Source: CAD feature listing. Evaluate the final solid. Frame: model axes, mm. Face numbers are marked on the shaded views. A direction names the side the tool comes from. Round coordinates to 2 decimals unless told otherwise and drop trailing zeros. Loops run counter-clockwise (first coordinate to the right, second up) from the corner with the lowest first, then second, coordinate; pieces in that order, holes last. Notation, with made-up numbers: (85, 41.25) - (128, 41.25) arc R9 ccw to (128, 45.25) - close; hole circle Ø2 at (23.25, 9). An arc over 180 degrees is marked (long way). One line per question, with ' | ' between items.
from build123d import *


with BuildPart() as part:
    # Skizze1 → Rotation1 (revolve)
    with BuildSketch(Plane.XY):
        with BuildLine():
            Line((0, 0), (-10, 0))
            Line((-10, 0), (-10, 2.4))
            Line((-10, 2.4), (-13.25, 2.4))
            ThreePointArc((-13.25, 2.4), (-16.785533906, 0.935533906), (-18.25, -2.6))
            Line((-18.25, -2.6), (-18.25, -5.85))
            Line((-18.25, -5.85), (-2.7, -5.85))
            Line((-2.7, -5.85), (-2.7, -0.8))
            Line((-2.7, -0.8), (0, -0.8))
            Line((0, -0.8), (0, 0))
        make_face()
    revolve(axis=Axis((-27.302993085, -5.85, 0), (1, 0, 0)))


solid = part.part
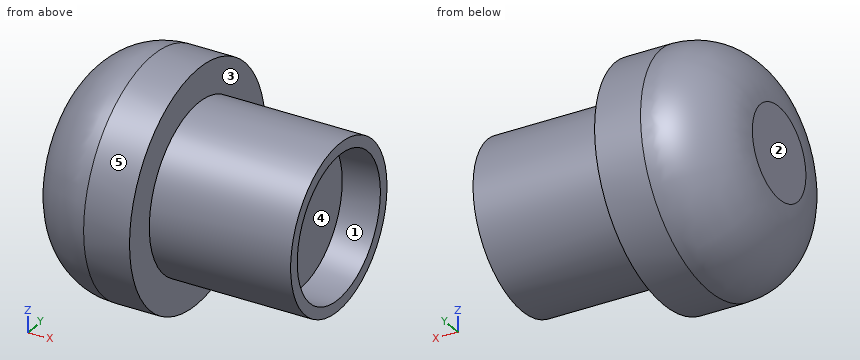
1. Access query for the marked faces 1 and 2. Directions: +Z, -Z, +X, -X, +Y, -Y. A direction counts if a zero-diameter tool reaches every point of the face in a straight line with its end or side. Return the directions, or none.
Worked out:
face 1: +X | face 2: +Z, -Z, -X, +Y, -Y
2. Material intervals for probe 1 along Z at (x, y) = (-1.9, -5.85); probe 2 along X at (y, z) = (-8, 2); probe 3 along Z at (x, y) = (-2.5, -10.25), sorted ascending.
Worked out:
probe 1: z = -5.85 to -5.05, 5.05 to 5.85 | probe 2: x = -18.25 to -2.7 | probe 3: z = -3.86 to -2.48, 2.48 to 3.86
3. Section query B-B, the plane x = -8. Return loops of the section in (y, z).
Worked out:
outline: circle Ø11.7 at (-5.85, 0)
4. Section query A-A, the plane x = -13. Return loops of the section in (y, z), plus the area to 3 significant figures.
Worked out:
outline: circle Ø16.5 at (-5.85, 0) | area: 214 mm2
5. Contact query for flat-ended pins moving along their axis: P1, Ø3, axis at y = -7.5, z = 6.5, coming from the -X side; P2, Ø3, axis at y = -5.5, z = -1, coming from the +X side; P3, Ø1, axis at x = -8.5, y = -10, coming from the +Z side. Output: stop coordinate, or through.
Worked out:
P1: stops at x = -17.85 | P2: stops at x = -2.7 | P3: stops at z = 4.57
6. Mould query, pull axis Z, two halves, no side actions, for the marked faces 3, 4 and 5. Classes: released by +Z, released by -Z, zero draft, split by the parting line, or undercut.
Worked out:
face 3: zero draft | face 4: undercut | face 5: split by the parting line
